from build123d import *

# Parameters (mm, degrees)
F1_DEPTH = 101.6


with BuildPart() as f1:
    # F0 (on Front) → F1 (new body)
    with BuildSketch(Plane.XZ):
        Polygon((0, 6), (0, 0), (19.5, 0), (19.5, 6), (16.5, 6), (16.5, 1.62), (3, 1.62), (3, 6), align=None)
        Polygon((3, 14.35), (3, 6), (3, 1.62), (16.5, 1.62), (16.5, 6), (16.5, 14.35), align=None)
    extrude(amount=F1_DEPTH)


solid = f1.part
Model file for the job. Use its own axes, mm. A direction names the side the tool comes from. Give positions to 0.01 mm unless a question says otherwise; leave off trailing zeros. Loops run counter-clockwise (first coordinate to the right, second up) from the corner with the lowest first, then second, coordinate; pieces in that order, holes last.
Item 1: Slice it at A-A (y = -41.5). Write the cut outline in (x, z), plus the area to 3 significant figures.
Check values:
outline: (0, 0) - (19.5, 0) - (19.5, 6) - (16.5, 6) - (16.5, 14.35) - (3, 14.35) - (3, 6) - (0, 6) - close
area: 230 mm2
Item 2: Slice it at C-C (z = 10). Write the cut outline in (x, y).
Check values:
outline: (3, -101.6) - (16.5, -101.6) - (16.5, 0) - (3, 0) - close
Item 3: Drill centre lines: line 1 along X through (y, z) = (-77, 11.25); line 2 along Z through (x, y) = (1.5, -33). Where is each one in solid material? Low to high.
Check values:
line 1: x = 3 to 16.5
line 2: z = 0 to 6
Item 4: Which spindle directions (+Z, -Z, +X, -X, +Y, -Y) get a long thin tool onto all of the face, cutting with end or side? Do faces 1 (the face through (2, -50, 6)), 2 (the face through (10, -50, 0)), 3 (the face through (16.5, -50, 10)). Say none if no direction does.
Check values:
face 1: +Z, -X, +Y, -Y
face 2: -Z, +X, -X, +Y, -Y
face 3: +Z, +X, +Y, -Y
Item 5: Drop flat-ended pins along their axis: P1, Ø1.5, axis at x = 17.5, y = -45, coming from the +Z side; P2, Ø2.5, axis at y = -55.5, z = 12, coming from the +X side. Give the stop position or say it passes through.
Check values:
P1: stops at z = 6
P2: stops at x = 16.5
Item 6: Slice it at B-B (x = 1.5). Write the cut outline in (y, z).
Check values:
outline: (-101.6, 0) - (0, 0) - (0, 6) - (-101.6, 6) - close
